Design review of the part shown in the three views and the two pictorial views. Dimensions are in mm from the part's minimum x, y and z. Round coordinates to 2 decimals unless told otherwise and drop trailing zeros. Loops run counter-clockwise (first coordinate to the right, second up) from the corner with the lowest first, then second, coordinate; pieces in that order, holes last.
1. Consider section C-C on z = 1.5. State the section outline as (x, y) points, then the cut area to 3 significant figures.
2. Consider section B-B on y = 50. State the section outline as (x, z) points.
3. To check wall thickness, follow line 1 along Y through (x, z) = (50, 3.05); line 2 along X through (y, z) = (80.5, 4.2); line 3 along X through (y, z) = (53, 4.35). State the ranges of each line that lie inside material, in increasing order.
4. Consider section D-D on y = 79.5. State the section outline as (x, z) points, then the cut area to 3 significant figures.
5. Consider section A-A on x = 50. State the section outline as (y, z) points, then the cut area to 3 significant figures.
6. Clearance check with flat-ended pins moving along their axes: pin 1 Ø1.5 at (x, z) = (68.5, 1) entering from +Y; pin 2 Ø3 at (x, z) = (92, 2) entering from -Y; pin 3 Ø3 at (y, z) = (76, 4) entering from -X. State where each tip first meets the part, or that it passes through.
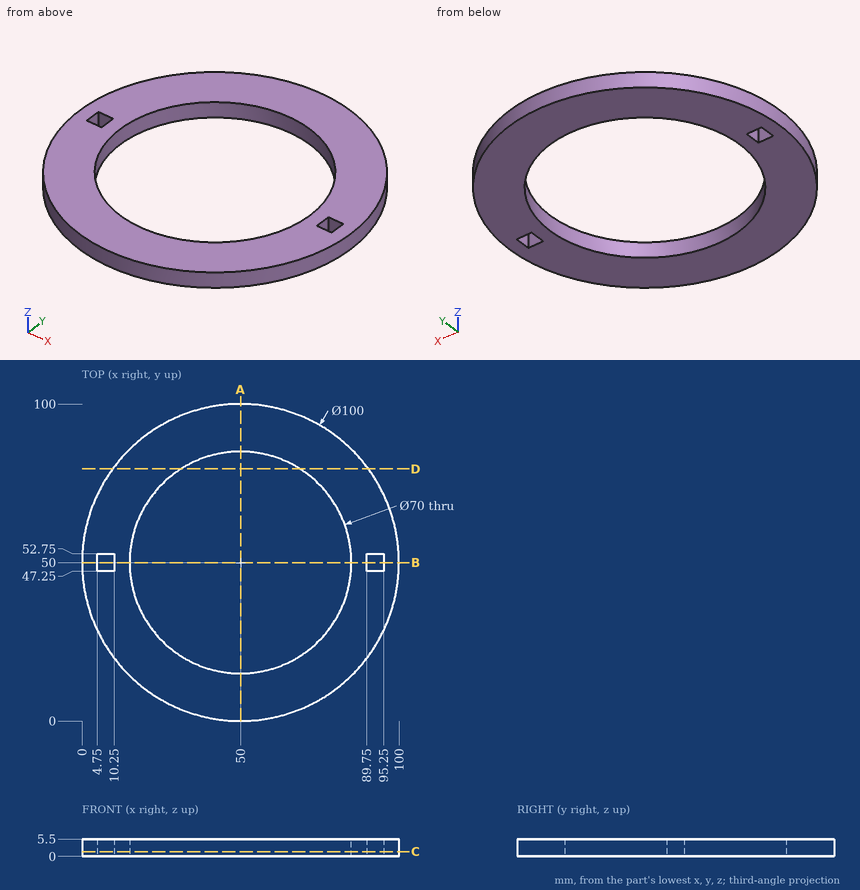
Resolved:
1. outline: circle Ø100 at (50, 50); hole (4.75, 47.25) - (10.25, 47.25) - (10.25, 52.75) - (4.75, 52.75) - close; hole circle Ø70 at (50, 50); hole (89.75, 47.25) - (95.25, 47.25) - (95.25, 52.75) - (89.75, 52.75) - close
1. area: 3,950 mm2
2. outline: (0, 0) - (4.75, 0) - (4.75, 5.5) - (0, 5.5) - close; (10.25, 0) - (15, 0) - (15, 5.5) - (10.25, 5.5) - close; (85, 0) - (89.75, 0) - (89.75, 5.5) - (85, 5.5) - close; (95.25, 0) - (100, 0) - (100, 5.5) - (95.25, 5.5) - close
3. line 1: y = 0 to 15, 85 to 100
3. line 2: x = 10.38 to 32.83, 67.17 to 89.62
3. line 3: x = 0.09 to 15.13, 84.87 to 99.91
4. outline: (9.63, 0) - (31.17, 0) - (31.17, 5.5) - (9.63, 5.5) - close; (68.83, 0) - (90.37, 0) - (90.37, 5.5) - (68.83, 5.5) - close
4. area: 237 mm2
5. outline: (0, 0) - (15, 0) - (15, 5.5) - (0, 5.5) - close; (85, 0) - (100, 0) - (100, 5.5) - (85, 5.5) - close
5. area: 165 mm2
6. pin 1: stops at y = 96.74
6. pin 2: stops at y = 20.68
6. pin 3: stops at x = 6.41
